Geometry check sheet. Reference: the model listing, model coordinates, mm. A direction names the side the tool comes from. Coordinates: 2 decimals unless noted, no trailing zeros. Write each loop counter-clockwise with the first axis right and the second up, starting at its lowest first coordinate (ties: lowest second). Pieces come first, ordered by that corner, then holes. Notation, with made-up numbers: (-23, 38) -> (21, 38) arc R26 cw to (21, 70) -> close; hole circle Ø6 at (67.5, -34). An arc over 180 degrees is marked (long way). Answer in a Markdown table with one row per item. Add a question column.
Q1. Gauge pin test, flat ends, axial feed: P1, Ø6.5, axis at x = 18, z = -12, coming from the -Y side; P2, Ø3.5, axis at x = 112.5, z = -1, coming from the +Y side; P3, Ø4, axis at x = 144, z = -11.5, coming from the +Y side; P4, Ø4, axis at y = 81, z = -14, coming from the -X side. Record the tip position at first contact, or that the pin passes through.
Q2. Tool access check on faces 4 (the face through (117, -4, -12)), 5 (the face through (117, 67, -3)), 6 (the face through (117, -1, -12)). Record the directions out of +Z, -Z, +X, -X, +Y, -Y that give a thin tool (end or side, any length) a straight path to the whole face; none if there is none.
Q3. Release check for a two-part mould opening along X. For faces 1 (the face through (117, 67, 0)), 2 (the face through (108.54, 78.224, -1.521)), 3 (the face through (33.27, 135.97, -1.14)) record: pulls with the +X half, pulls with the -X half, needs draft (parallel to the pull), parting line crosses it, or undercut.
Q4. Thickness scan on line 1 (X direction, y = -3.3, z = -12); line 2 (Y direction, x = 132, z = -6.5); line 3 (Z direction, x = 105, y = 196.5). Record the ranges inside material, lowest first.
Q5. Section check A-A, the plane x = 115. Record the boundary of the cut face in (y, z), and give its area (3 significant figures).
```python
from build123d import *

# Parameters (mm, degrees)
SKETCH_10_R                   = 10
SM_BASE_FLANGE_3_DEPTH        = 3
SM_EDGE_FLANGE_6_DEPTH        = 230
SM_EDGE_FLANGE_6_BEND_DEPTH   = 230
SM_EDGE_FLANGE_6_BEND_2_DEPTH = 230
CUT_EXTRUDE_4_REACH           = 364.518
SKETCH_47_R                   = 2
CUT_EXTRUDE_6_REACH           = 265.651
SKETCH_50_R                   = 2
CUT_EXTRUDE_7_REACH           = 353.429
SKETCH_51_R                   = 2
CUT_EXTRUDE_8_REACH           = 350.533
SKETCH_52_R                   = 14


# Sheet-metal steps are written as plain solids
with BuildPart() as part:
    # Эскиз10 → Базовая кромка3 (new body)
    with BuildSketch(Plane.XY):
        Polygon((0, 0), (-21, 36.373066959), (94, 235.558909829), (136, 235.558909829), (251, 36.373066959), (230, 0), align=None)
        with Locations((171.849364905, 123.465988394)):
            Circle(SKETCH_10_R, mode=Mode.SUBTRACT)
    extrude(amount=-SM_BASE_FLANGE_3_DEPTH)

    # Ребро-кромка6 section (across the edge) → Ребро-кромка6 (add)
    with BuildSketch(Plane(origin=(-21.866025404, 36.873066959, -3), x_dir=(0.8660254037844436, -0.4999999999999914, -3.4914813388431334e-15), z_dir=(0.4999999999999914, 0.8660254037844436, 0))):
        with BuildLine():
            Line((-3, 1), (-3, 17))
            Line((-3, 17), (0, 17))
            Line((0, 17), (0, 1))
            ThreePointArc((0, 1), (0.292893219, 0.292893219), (1, 0))
            Line((1, 0), (1, -3))
            ThreePointArc((1, -3), (-1.828427125, -1.828427125), (-3, 1))
        make_face()
    extrude(amount=SM_EDGE_FLANGE_6_DEPTH)

    # Ребро-кромка6 section 2 (across the edge) → Ребро-кромка6 bend (add)
    with BuildSketch(Plane(origin=(136.866025404, 236.058909829, -3), x_dir=(-0.8660254037844363, -0.5000000000000041, -3.4914813388431334e-15), z_dir=(0.5000000000000041, -0.8660254037844363, 0))):
        with BuildLine():
            Line((-3, 1), (-3, 17))
            Line((-3, 17), (0, 17))
            Line((0, 17), (0, 1))
            ThreePointArc((0, 1), (0.292893219, 0.292893219), (1, 0))
            Line((1, 0), (1, -3))
            ThreePointArc((1, -3), (-1.828427125, -1.828427125), (-3, 1))
        make_face()
    extrude(amount=SM_EDGE_FLANGE_6_BEND_DEPTH)

    # Ребро-кромка6 section 3 (across the edge) → Ребро-кромка6 bend 2 (add)
    with BuildSketch(Plane(origin=(230, -1, -3), x_dir=(0, 1, 0), z_dir=(-1, 0, 0))):
        with BuildLine():
            Line((-3, 1), (-3, 17))
            Line((-3, 17), (0, 17))
            Line((0, 17), (0, 1))
            ThreePointArc((0, 1), (0.292893219, 0.292893219), (1, 0))
            Line((1, 0), (1, -3))
            ThreePointArc((1, -3), (-1.828427125, -1.828427125), (-3, 1))
        make_face()
    extrude(amount=SM_EDGE_FLANGE_6_BEND_2_DEPTH)

    # Эскиз47 → Вырез-Вытянуть4 (cut, up to next)
    with BuildSketch(Plane(origin=(-34.964101615, 20.186533479, 0), x_dir=(0, 0, 1), z_dir=(-0.866025403784443, 0.4999999999999925, 3.788649256556814e-15)), mode=Mode.PRIVATE) as cut_extrude_4_sk1:
        with Locations(Location((-12, 29, 0), (0, 0, 270))):
            Circle(SKETCH_47_R)
    cut_extrude_4_tool1 = extrude(cut_extrude_4_sk1.sketch, amount=-CUT_EXTRUDE_4_REACH, mode=Mode.PRIVATE) & part.part
    # Эскиз47 → Вырез-Вытянуть4 (cut, up to next)
    with BuildSketch(Plane(origin=(-34.964101615, 20.186533479, 0), x_dir=(0, 0, 1), z_dir=(-0.866025403784443, 0.4999999999999925, 3.788649256556814e-15)), mode=Mode.PRIVATE) as cut_extrude_4_sk2:
        with Locations(Location((-12, 39, 0), (0, 0, 270))):
            Circle(SKETCH_47_R)
    cut_extrude_4_tool2 = extrude(cut_extrude_4_sk2.sketch, amount=-CUT_EXTRUDE_4_REACH, mode=Mode.PRIVATE) & part.part
    # Эскиз47 → Вырез-Вытянуть4 (cut, up to next)
    with BuildSketch(Plane(origin=(-34.964101615, 20.186533479, 0), x_dir=(0, 0, 1), z_dir=(-0.866025403784443, 0.4999999999999925, 3.788649256556814e-15)), mode=Mode.PRIVATE) as cut_extrude_4_sk3:
        with Locations(Location((-12, 233, 0), (0, 0, 270))):
            Circle(SKETCH_47_R)
    cut_extrude_4_tool3 = extrude(cut_extrude_4_sk3.sketch, amount=-CUT_EXTRUDE_4_REACH, mode=Mode.PRIVATE) & part.part
    # Эскиз47 → Вырез-Вытянуть4 (cut, up to next)
    with BuildSketch(Plane(origin=(-34.964101615, 20.186533479, 0), x_dir=(0, 0, 1), z_dir=(-0.866025403784443, 0.4999999999999925, 3.788649256556814e-15)), mode=Mode.PRIVATE) as cut_extrude_4_sk4:
        with Locations(Location((-12, 243, 0), (0, 0, 270))):
            Circle(SKETCH_47_R)
    cut_extrude_4_tool4 = extrude(cut_extrude_4_sk4.sketch, amount=-CUT_EXTRUDE_4_REACH, mode=Mode.PRIVATE) & part.part
    add(cut_extrude_4_tool1.solids().sort_by_distance((-20.464102, 45.30127, -12))[0], mode=Mode.SUBTRACT)
    add(cut_extrude_4_tool2.solids().sort_by_distance((-15.464102, 53.961524, -12))[0], mode=Mode.SUBTRACT)
    add(cut_extrude_4_tool3.solids().sort_by_distance((81.535898, 221.970453, -12))[0], mode=Mode.SUBTRACT)
    add(cut_extrude_4_tool4.solids().sort_by_distance((86.535898, 230.630707, -12))[0], mode=Mode.SUBTRACT)

    # Эскиз50 → Вырез-Вытянуть6 (cut, up to next)
    with BuildSketch(Plane(origin=(207.464101615, 119.779454915, 0), x_dir=(0, 0, -1), z_dir=(0.866025403784436, 0.5000000000000047, 3.0623287353932815e-15)), mode=Mode.PRIVATE) as cut_extrude_6_sk1:
        with Locations(Location((12, -86, 0), (0, 0, 90))):
            Circle(SKETCH_50_R)
    cut_extrude_6_tool1 = extrude(cut_extrude_6_sk1.sketch, amount=-CUT_EXTRUDE_6_REACH, mode=Mode.PRIVATE) & part.part
    # Эскиз50 → Вырез-Вытянуть6 (cut, up to next)
    with BuildSketch(Plane(origin=(207.464101615, 119.779454915, 0), x_dir=(0, 0, -1), z_dir=(0.866025403784436, 0.5000000000000047, 3.0623287353932815e-15)), mode=Mode.PRIVATE) as cut_extrude_6_sk2:
        with Locations(Location((12, -76, 0), (0, 0, 90))):
            Circle(SKETCH_50_R)
    cut_extrude_6_tool2 = extrude(cut_extrude_6_sk2.sketch, amount=-CUT_EXTRUDE_6_REACH, mode=Mode.PRIVATE) & part.part
    # Эскиз50 → Вырез-Вытянуть6 (cut, up to next)
    with BuildSketch(Plane(origin=(207.464101615, 119.779454915, 0), x_dir=(0, 0, -1), z_dir=(0.866025403784436, 0.5000000000000047, 3.0623287353932815e-15)), mode=Mode.PRIVATE) as cut_extrude_6_sk3:
        with Locations(Location((12, 118, 0), (0, 0, 90))):
            Circle(SKETCH_50_R)
    cut_extrude_6_tool3 = extrude(cut_extrude_6_sk3.sketch, amount=-CUT_EXTRUDE_6_REACH, mode=Mode.PRIVATE) & part.part
    # Эскиз50 → Вырез-Вытянуть6 (cut, up to next)
    with BuildSketch(Plane(origin=(207.464101615, 119.779454915, 0), x_dir=(0, 0, -1), z_dir=(0.866025403784436, 0.5000000000000047, 3.0623287353932815e-15)), mode=Mode.PRIVATE) as cut_extrude_6_sk4:
        with Locations(Location((12, 128, 0), (0, 0, 90))):
            Circle(SKETCH_50_R)
    cut_extrude_6_tool4 = extrude(cut_extrude_6_sk4.sketch, amount=-CUT_EXTRUDE_6_REACH, mode=Mode.PRIVATE) & part.part
    add(cut_extrude_6_tool1.solids().sort_by_distance((250.464102, 45.30127, -12))[0], mode=Mode.SUBTRACT)
    add(cut_extrude_6_tool2.solids().sort_by_distance((245.464102, 53.961524, -12))[0], mode=Mode.SUBTRACT)
    add(cut_extrude_6_tool3.solids().sort_by_distance((148.464102, 221.970453, -12))[0], mode=Mode.SUBTRACT)
    add(cut_extrude_6_tool4.solids().sort_by_distance((143.464102, 230.630707, -12))[0], mode=Mode.SUBTRACT)

    # Эскиз51 → Вырез-Вытянуть7 (cut, up to next)
    with BuildSketch(Plane.XZ.offset(4), mode=Mode.PRIVATE) as cut_extrude_7_sk1:
        with Locations(Location((222, -12, 0), (0, 0, 270))):
            Circle(SKETCH_51_R)
    cut_extrude_7_tool1 = extrude(cut_extrude_7_sk1.sketch, amount=-CUT_EXTRUDE_7_REACH, mode=Mode.PRIVATE) & part.part
    # Эскиз51 → Вырез-Вытянуть7 (cut, up to next)
    with BuildSketch(Plane.XZ.offset(4), mode=Mode.PRIVATE) as cut_extrude_7_sk2:
        with Locations(Location((212, -12, 0), (0, 0, 270))):
            Circle(SKETCH_51_R)
    cut_extrude_7_tool2 = extrude(cut_extrude_7_sk2.sketch, amount=-CUT_EXTRUDE_7_REACH, mode=Mode.PRIVATE) & part.part
    # Эскиз51 → Вырез-Вытянуть7 (cut, up to next)
    with BuildSketch(Plane.XZ.offset(4), mode=Mode.PRIVATE) as cut_extrude_7_sk3:
        with Locations(Location((18, -12, 0), (0, 0, 270))):
            Circle(SKETCH_51_R)
    cut_extrude_7_tool3 = extrude(cut_extrude_7_sk3.sketch, amount=-CUT_EXTRUDE_7_REACH, mode=Mode.PRIVATE) & part.part
    # Эскиз51 → Вырез-Вытянуть7 (cut, up to next)
    with BuildSketch(Plane.XZ.offset(4), mode=Mode.PRIVATE) as cut_extrude_7_sk4:
        with Locations(Location((8, -12, 0), (0, 0, 270))):
            Circle(SKETCH_51_R)
    cut_extrude_7_tool4 = extrude(cut_extrude_7_sk4.sketch, amount=-CUT_EXTRUDE_7_REACH, mode=Mode.PRIVATE) & part.part
    add(cut_extrude_7_tool1.solids().sort_by_distance((222, -4, -12))[0], mode=Mode.SUBTRACT)
    add(cut_extrude_7_tool2.solids().sort_by_distance((212, -4, -12))[0], mode=Mode.SUBTRACT)
    add(cut_extrude_7_tool3.solids().sort_by_distance((18, -4, -12))[0], mode=Mode.SUBTRACT)
    add(cut_extrude_7_tool4.solids().sort_by_distance((8, -4, -12))[0], mode=Mode.SUBTRACT)

    # Эскиз52 → Вырез-Вытянуть8 (cut, up to next)
    with BuildSketch(Plane(origin=(0, 0, -3), x_dir=(-1, 0, 0), z_dir=(0, 0, -1)), mode=Mode.PRIVATE) as cut_extrude_8_sk1:
        with Locations((-115, 90.643992263)):
            Circle(SKETCH_52_R)
    cut_extrude_8_tool1 = extrude(cut_extrude_8_sk1.sketch, amount=-CUT_EXTRUDE_8_REACH, mode=Mode.PRIVATE) & part.part
    add(cut_extrude_8_tool1.solids().sort_by_distance((115, 90.643992, -3))[0], mode=Mode.SUBTRACT)


solid = part.part
```
Calculated:
| question | item | result |
|---|---|---|
| 1 | P1 | stops at y = -4 |
| 1 | P2 | stops at y = 235.56 |
| 1 | P3 | stops at y = 233.17 |
| 1 | P4 | stops at x = -1.01 |
| 2 | face 4 | +Z, -Z, +X, -X, -Y |
| 2 | face 5 | -Z |
| 2 | face 6 | -Z, +X, -X |
| 3 | face 1 | needs draft |
| 3 | face 2 | undercut |
| 3 | face 3 | pulls with the -X half |
| 4 | line 1 | x = 0 to 6, 10 to 16, 20 to 210, 214 to 220, 224 to 230 |
| 4 | line 2 | y = -4 to -1 |
| 4 | line 3 | z = -3 to 0 |
| 5 | outline | (-4, -20) -> (-1, -20) -> (-1, -4) arc R1 cw to (0, -3) -> (76.64, -3) -> (76.64, 0) -> (0, 0) arc R4 ccw to (-4, -4) -> close; (104.64, -3) -> (235.56, -3) -> (235.56, 0) -> (104.64, 0) -> close |
| 5 | area | 682 mm² |
